Source: CAD feature listing. Evaluate the final solid. Frame: model axes, mm. A direction names the side the tool comes from. Give positions to 0.01 mm unless a question says otherwise; leave off trailing zeros. Loops run counter-clockwise (first coordinate to the right, second up) from the corner with the lowest first, then second, coordinate; pieces in that order, holes last. Notation, with made-up numbers: (35, 23) -> (47, 23) arc R21 ccw to (47, 29) -> close; hole circle Ø6 at (9, 22.5). An arc over 180 degrees is marked (long way). Answer as a JSON object with one key per item and string values. Group by question number.
from build123d import *

# Parameters (mm, degrees)
BOSS_EXTRUDE1_DEPTH = 5
CAVITY1_OUTLINE_R   = 0.85
CAVITY1_OUTLINE_R_2 = 7.5
CAVITY1_DEPTH       = 5


# Read off the part's stored shape, not the designer's step: Cavity1
with BuildPart() as part:
    # Sketch1 → Boss-Extrude1 (new body)
    with BuildSketch(Plane.XY):
        Polygon((-25.25, 7.5), (-25.25, 22.5), (-10.25, 22.5), (-10.25, 27.5), (4.75, 27.5), (4.75, 22.5), (19.75, 22.5), (19.75, 7.5), (24.75, 7.5), (24.75, -7.5), (19.75, -7.5), (19.75, -22.5), (4.75, -22.5), (4.75, -27.5), (-10.25, -27.5), (-10.25, -22.5), (-25.25, -22.5), (-25.25, -7.5), (-30.25, -7.5), (-30.25, 7.5), align=None)
    extrude(amount=BOSS_EXTRUDE1_DEPTH)

    # Cavity1 outline → Cavity1 (cut)
    with BuildSketch(Plane.XY):
        with Locations((2.325, 8.790157848)):
            Circle(CAVITY1_OUTLINE_R)
        with Locations((-7.825, 8.790157848)):
            Circle(CAVITY1_OUTLINE_R)
        with Locations((-12.9, 0)):
            Circle(CAVITY1_OUTLINE_R)
        with Locations((-7.825, -8.790157848)):
            Circle(CAVITY1_OUTLINE_R)
        with Locations((2.325, -8.790157848)):
            Circle(CAVITY1_OUTLINE_R)
        with Locations((7.4, 0)):
            Circle(CAVITY1_OUTLINE_R)
        with Locations((-2.75, 0)):
            Circle(CAVITY1_OUTLINE_R_2)
    extrude(amount=CAVITY1_DEPTH, mode=Mode.SUBTRACT)


solid = part.part
(1) Mould query, pull axis Y, two halves, no side actions, for faces 1 (the face through (19.75, -15, 2)), 2 (the face through (12, -22.5, 2)), 3 (the face through (-12.09, 0.26, 2.46)), 4 (the face through (2.14, -9.62, 2.46)). Classes: pulls with the +Y half, pulls with the -Y half, needs draft (parallel to the pull), parting line crosses it, or undercut.
(2) Access query for faces 5 (the face through (4.75, -25, 2)), 6 (the face through (4, 6, 0)), 7 (the face through (12, 22.5, 2)), 8 (the face through (-25.25, -15, 2)), 9 (the face through (-18, 22.5, 2)). Directions: +Z, -Z, +X, -X, +Y, -Y. A direction counts if a zero-diameter tool reaches every point of the face in a straight line with its end or side. Return the directions, or none.
(3) Section query C-C on z = 4.35. Return the cut outline in (x, y) (3 decimals).
(4) First-contact query: pin 1 (2.5 mm diameter, centred on x = -12.9, y = 0, fed in from +Z); pin 2 (3 mm diameter, centred on x = 14, z = 4.5, fed in from -Y); pin 3 (1.5 mm diameter, centred on x = -28.5, z = 3, fed in from -Y); pin 4 (1.5 mm diameter, centred on y = 25.5, z = 3, fed in from -X). Flat tips, straight axial feed; report the tip coordinate or a pass-through.
(5) Section query A-A on y = 0. Return the cut outline in (x, z).
(6) Section query D-D on y = -6.5. Return the cut outline in (x, z).
(7) Material intervals for line 1 (Y direction, x = -13, z = 0.5); line 2 (Y direction, x = 14, z = 1.65); line 3 (Y direction, x = -4, z = 1.7), sorted ascending. Write a range as from..to.
(8) Section query B-B on x = 7.4. Return the cut outline in (y, z).
Result:
{
 "1": {"face 1": "needs draft", "face 2": "pulls with the -Y half", "face 3": "undercut", "face 4": "undercut"},
 "2": {"face 5": "+Z, -Z, +X, -Y", "face 6": "-Z, +X, -X, +Y, -Y", "face 7": "+Z, -Z, +X, +Y", "face 8": "+Z, -Z, -X, -Y", "face 9": "+Z, -Z, -X, +Y"},
 "3": {"outline": "(-30.25, -7.5) -> (-25.25, -7.5) -> (-25.25, -22.5) -> (-10.25, -22.5) -> (-10.25, -27.5) -> (4.75, -27.5) -> (4.75, -22.5) -> (19.75, -22.5) -> (19.75, -7.5) -> (24.75, -7.5) -> (24.75, 7.5) -> (19.75, 7.5) -> (19.75, 22.5) -> (4.75, 22.5) -> (4.75, 27.5) -> (-10.25, 27.5) -> (-10.25, 22.5) -> (-25.25, 22.5) -> (-25.25, 7.5) -> (-30.25, 7.5) -> close; hole circle Ø1.7 at (-12.9, 0); hole circle Ø15 at (-2.75, 0); hole circle Ø1.7 at (-7.825, -8.79); hole circle Ø1.7 at (-7.825, 8.79); hole circle Ø1.7 at (2.325, -8.79); hole circle Ø1.7 at (2.325, 8.79); hole circle Ø1.7 at (7.4, 0)"},
 "4": {"pin 1": "z = 5", "pin 2": "y = -22.5", "pin 3": "y = -7.5", "pin 4": "x = -10.25"},
 "5": {"outline": "(-30.25, 0) -> (-13.75, 0) -> (-13.75, 5) -> (-30.25, 5) -> close; (-12.05, 0) -> (-10.25, 0) -> (-10.25, 5) -> (-12.05, 5) -> close; (4.75, 0) -> (6.55, 0) -> (6.55, 5) -> (4.75, 5) -> close; (8.25, 0) -> (24.75, 0) -> (24.75, 5) -> (8.25, 5) -> close"},
 "6": {"outline": "(-30.25, 0) -> (-6.49, 0) -> (-6.49, 5) -> (-30.25, 5) -> close; (0.99, 0) -> (24.75, 0) -> (24.75, 5) -> (0.99, 5) -> close"},
 "7": {"line 1": "-22.5..-0.84, 0.84..22.5", "line 2": "-22.5..22.5", "line 3": "-27.5..-7.4, 7.4..27.5"},
 "8": {"outline": "(-22.5, 0) -> (-0.85, 0) -> (-0.85, 5) -> (-22.5, 5) -> close; (0.85, 0) -> (22.5, 0) -> (22.5, 5) -> (0.85, 5) -> close"}
}
